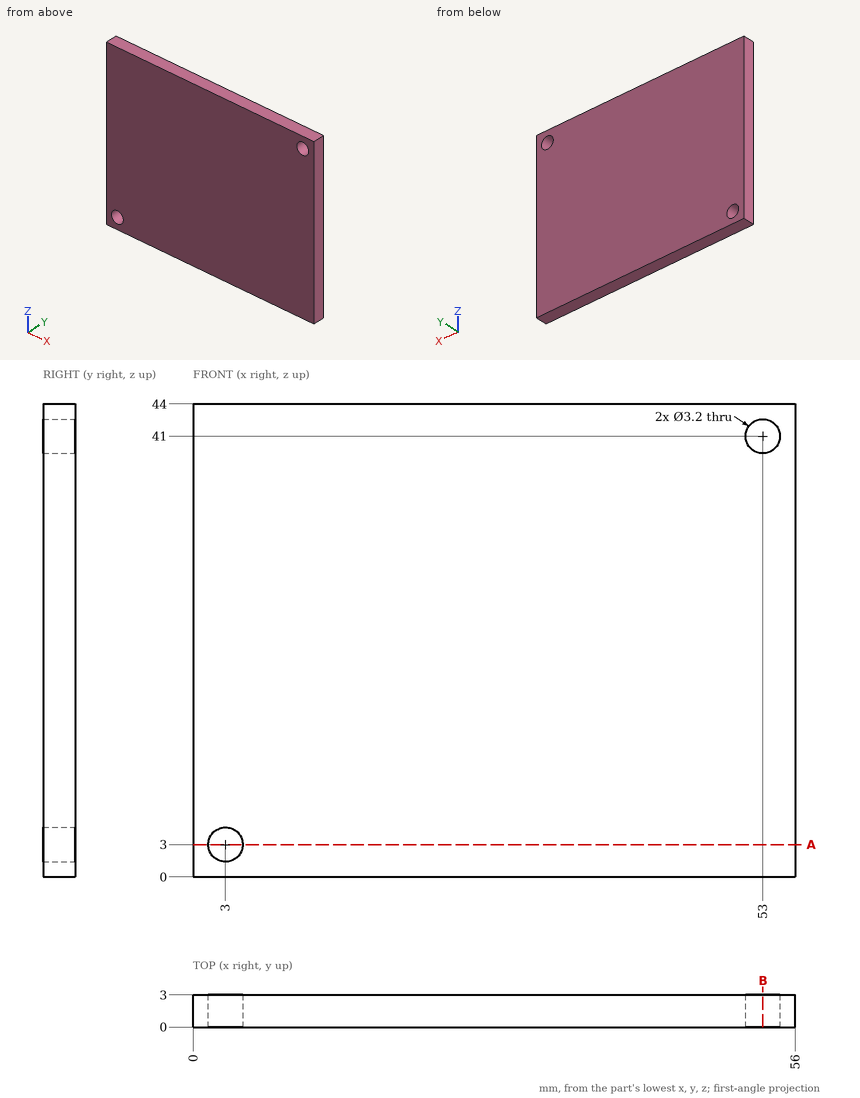
Geometry: see drawing. Coordinates: mm, zero at the bounding-box minimum. Coordinates: 2 decimals unless noted, no trailing zeros. Order: outer loops, then holes, each group sorted by start corner. A loop starts at its lowest first (then second) coordinate and runs counter-clockwise, first axis right, second up. Notation, with made-up numbers: M 15,35.25 L 40,35.25 A22 ccw 40,74.25 Z; hole C 52.5,5 d7. An arc over 180 degrees is marked long. Write item = value, one per line. Start each with the question number.
(1) Section A-A on z = 3. Output: boundary loops of the cut face in (x, y).
(2) First-contact query: P1, Ø1.9, axis at x = 53, z = 41, coming from the -Y side. Flat tip, straight axial feed; report the tip coordinate or a pass-through.
(3) Section B-B on x = 53. Output: boundary loops of the cut face in (y, z).
(4) Line query: line 1 along X through (y, z) = (0.85, 3); line 2 along Z through (x, y) = (53, 2.2); line 3 along X through (y, z) = (1.25, 41). Output: solid intervals per line, ascending. Write a range as [from, to].
Result set:
q1.outline = M 0,0 L 1.4,0 L 1.4,3 L 0,3 Z; M 4.6,0 L 56,0 L 56,3 L 4.6,3 Z
q2.P1 = through
q3.outline = M 0,0 L 3,0 L 3,39.4 L 0,39.4 Z; M 0,42.6 L 3,42.6 L 3,44 L 0,44 Z
q4.line_1 = [0, 1.4], [4.6, 56]
q4.line_2 = [0, 39.4], [42.6, 44]
q4.line_3 = [0, 51.4], [54.6, 56]
